```python
from build123d import *

# Parameters (mm, degrees)
SKETCH002_R          = 80
SKETCH003_R          = 24.3
SKETCH004_R          = 24.3
PAD001_DEPTH         = 105
SKETCH005_R          = 22.7
SKETCH006_R          = 77.5
SKETCH011_R          = 22.7
POCKET001_DEPTH      = 5
POCKET001_DEPTH_BACK = 100
SKETCH008_R          = 22.7
POCKET002_DEPTH      = 5
SKETCH009_R          = 24.3
SKETCH009_R_2        = 22.7
PAD002_DEPTH         = 28
SKETCH010_W          = 8
SKETCH010_H          = 2.54
POCKET003_DEPTH      = 100
POCKET003_DEPTH_BACK = 100
SKETCH_R             = 24.3
SKETCH_R_2           = 22.7
PAD_DEPTH            = 29
SKETCH001_W          = 8
SKETCH001_H          = 2.6
POCKET_DEPTH         = 100
POCKET_DEPTH_BACK    = 100
PAD003_DEPTH         = 0.8
PAD003_DEPTH_BACK    = 0.8
POLARPATTERN_COUNT   = 4


with BuildPart() as body001:
    # Sketch002 → AdditiveLoft section 0
    with BuildSketch(Plane.XY):
        Circle(SKETCH002_R)
    # Sketch003 → AdditiveLoft section 1
    with BuildSketch(Plane.XY.offset(150)):
        Circle(SKETCH003_R)
    loft()

    # Sketch004 → Pad001 (new body)
    with BuildSketch(Plane.XZ):
        with Locations((44, 26)):
            Circle(SKETCH004_R)
    extrude(amount=PAD001_DEPTH)

    # Sketch005 (on Face3 of Pad001) → SubtractiveLoft section 0
    with BuildSketch(Plane.XY.offset(150)):
        Circle(SKETCH005_R)
    # Sketch006 (on Face1 of Pad001) → SubtractiveLoft section 1
    with BuildSketch(Plane(origin=(0, 0, 3), x_dir=(1, 0, 0), z_dir=(0, 0, -1))):
        Circle(SKETCH006_R)
    loft(mode=Mode.SUBTRACT)

    # Sketch011 → Pocket001 (cut, two sides)
    with BuildSketch(Plane.XZ.offset(12)) as pocket001_sk:
        with Locations((44, 26)):
            Circle(SKETCH011_R)
    extrude(amount=-POCKET001_DEPTH, mode=Mode.SUBTRACT)
    extrude(pocket001_sk.sketch, amount=POCKET001_DEPTH_BACK, mode=Mode.SUBTRACT)

    # Sketch008 → Pocket002 (cut)
    with BuildSketch(Plane.XY):
        Circle(SKETCH008_R)
    extrude(amount=POCKET002_DEPTH, mode=Mode.SUBTRACT)

    # Sketch009 → Pad002 (join)
    with BuildSketch(Plane.XY.offset(150)):
        Circle(SKETCH009_R)
        Circle(SKETCH009_R_2, mode=Mode.SUBTRACT)
    extrude(amount=PAD002_DEPTH)

    # Sketch010 → Pocket003 (cut, two sides)
    with BuildSketch(Plane.YZ) as pocket003_sk:
        with Locations((0, 172.47)):
            Rectangle(SKETCH010_W, SKETCH010_H)
    extrude(amount=-POCKET003_DEPTH, mode=Mode.SUBTRACT)
    extrude(pocket003_sk.sketch, amount=POCKET003_DEPTH_BACK, mode=Mode.SUBTRACT)


with BuildPart() as body:
    # Sketch → Pad (new body)
    with BuildSketch(Plane.XY):
        Circle(SKETCH_R)
        Circle(SKETCH_R_2, mode=Mode.SUBTRACT)
    extrude(amount=PAD_DEPTH)

    # Sketch001 → Pocket (cut, two sides)
    with BuildSketch(Plane.XZ) as pocket_sk:
        with Locations((0, 26.3)):
            Rectangle(SKETCH001_W, SKETCH001_H)
    extrude(amount=-POCKET_DEPTH, mode=Mode.SUBTRACT)
    extrude(pocket_sk.sketch, amount=POCKET_DEPTH_BACK, mode=Mode.SUBTRACT)

    # Boolean: union Body001
    add(body001.part)

    # Sketch012 → Pad003 (join, two sides)
    with BuildSketch(Plane.XZ) as pad003_sk:
        Polygon((24.3, 29), (39.3, 0), (24.3, 0), align=None)
    pad003 = extrude(amount=PAD003_DEPTH) + extrude(pad003_sk.sketch, amount=-PAD003_DEPTH_BACK)

    # PolarPattern: Pad003 ×4 about axis
    polarpattern_axis = Axis((0, 0, 0), (0, 0, 1))
    for i in range(1, POLARPATTERN_COUNT):
        add(pad003.rotate(polarpattern_axis, i * 360 / POLARPATTERN_COUNT))


solid = body.part
```
CAD build for the part. Positions are in the model's coordinates, mm. A direction names the side the tool comes from. Round coordinates to 2 decimals unless told otherwise and drop trailing zeros. Order: outer loops, then holes, each group sorted by start corner. A loop starts at its lowest first (then second) coordinate and runs counter-clockwise, first axis right, second up.
Item 1: Saw through at A-A on y = -89. Write the cut outline in (x, z).
Item 2: Mould opens along Z. For faces 1 (the face through (17, -17, 0)), 2 (the face through (-0.8, 28, 10)), 3 (the face through (-7, 22, 178)) say: pulls with the +Z half, pulls with the -Z half, needs draft (parallel to the pull), parting line crosses it, or undercut.
Item 3: Saw through at B-B on z = 34. Write the cut outline in (x, y).
Item 4: Probe line 1 along Y through (x, z) = (0, 158.75); line 2 along X through (y, z) = (7, 25.5); line 3 along Y through (x, z) = (-6, 126.5). List the from-to ranges inside material, lowest first.
Item 5: Saw through at C-C on z = 141.5. Write the cut outline in (x, y), then the cut area to 3 significant figures.
Item 6: Tool access for faces 4 (the face through (10.47, -20.14, 14.3)), 5 (the face through (67.178, -77.238, 33.299)), 6 (the face through (16.993, -17.371, 15.818)): list every direction of +Z, -Z, +X, -X, +Y, -Y with a clear straight run to the whole face (end or side of a thin tool).
Item 7: Pin check, flat tips, straight feed: pin 1 (11 mm diameter, centred on y = -30, z = 22, fed in from +X); pin 2 (1.8 mm diameter, centred on y = -23.5, z = 26.5, fed in from +X); pin 3 (1.5 mm diameter, centred on y = 35.5, z = 89.5, fed in from -X). Stop position of each tip, or through.
Reported:
1. outline: circle Ø48.6 at (44, 26); hole circle Ø45.4 at (44, 26)
2. face 1: pulls with the -Z half
2. face 2: undercut
2. face 3: pulls with the +Z half
3. outline: (21.05, -105) - (22.76, -105) - (22.76, -61.89) arc R65.94 cw (long way) to (65.24, -9.58) - (65.24, -105) - (66.95, -105) - (66.95, -7.59) arc R67.37 ccw (long way) to (21.05, -64) - close
4. line 1: y = -24.3 to -22.7, 22.7 to 24.3
4. line 2: x = -70.18 to -68.76, -23.27 to -21.59, 21.59 to 23.27, 68.76 to 70.18
4. line 3: y = -32.48 to -30.88, 30.88 to 32.48
5. outline: circle Ø54.91 at (0, 0); hole circle Ø51.74 at (0, 0)
5. area: 266 mm2
6. face 4: +Z, -Z
6. face 5: -Y
6. face 6: none
7. pin 1: stops at x = 68.47
7. pin 2: stops at x = 68.3
7. pin 3: stops at x = -31.39
